Build history of the part. All positions in model axes, mm. Face numbers are marked on the shaded views. A direction names the side the tool comes from. Round coordinates to 2 decimals unless told otherwise and drop trailing zeros. Loops run counter-clockwise (first coordinate to the right, second up) from the corner with the lowest first, then second, coordinate; pieces in that order, holes last.
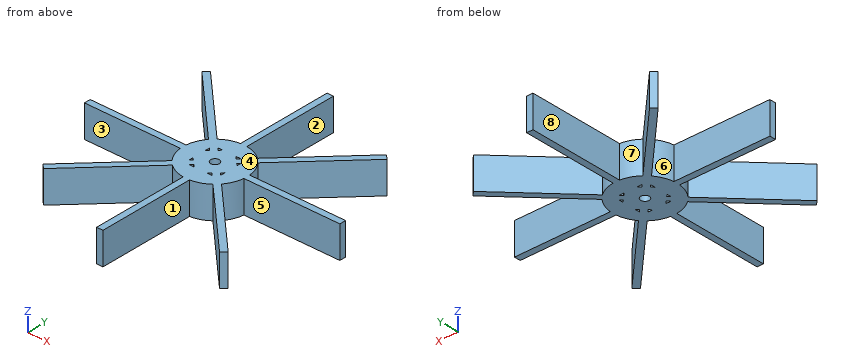
from build123d import *

# Parameters (mm, degrees)
F3_DEPTH = 10
F4_DEPTH = 10
F5_R     = 1.35
F6_DEPTH = 25


with BuildPart() as f3:
    # F2 (on Top) → F3 (new body)
    with BuildSketch(Plane.XY):
        Polygon((-2.9411380965, 1.5269245341), (-4.2426406871, 2.8284271247), (-7.0710678119, 0), (-5.7695652212, -1.3015025906), align=None)
        Polygon((-28.9913780286, 27.5771644663), (-4.2426406871, 2.8284271247), (-3.5355339059, 3.5355339059), (-2.8284271247, 4.2426406871), (-27.5771644663, 28.9913780286), align=None)
        Polygon((-3.5355339059, 3.5355339059), (-4.2426406871, 2.8284271247), (-2.9411380965, 1.5269245341), (-5.7695652212, -1.3015025906), (-4.2426406871, -2.8284271247), (-3.5355339059, -3.5355339059), (0, 0), align=None)
        Polygon((-2.8284271247, 4.2426406871), (-3.5355339059, 3.5355339059), (0, 0), (3.5355339059, 3.5355339059), (2.8284271247, 4.2426406871), (2.4045457253, 4.6665220865), (-0.4238813994, 1.8380949618), align=None)
        Polygon((0, 7.0710678119), (-2.8284271247, 4.2426406871), (-0.4238813994, 1.8380949618), (2.4045457253, 4.6665220865), align=None)
        Polygon((3.5355339059, 3.5355339059), (0, 0), (3.5355339059, -3.5355339059), (4.2426406871, -2.8284271247), (7.0710678119, 0), (4.2426406871, 2.8284271247), align=None)
        Polygon((3.5355339059, -3.5355339059), (0, 0), (-3.5355339059, -3.5355339059), (-2.8284271247, -4.2426406871), (0, -7.0710678119), (2.8284271247, -4.2426406871), align=None)
        Polygon((-3.5355339059, -3.5355339059), (-4.2426406871, -2.8284271247), (-28.9913780286, -27.5771644663), (-27.5771644663, -28.9913780286), (-2.8284271247, -4.2426406871), align=None)
        Polygon((4.2426406871, -2.8284271247), (3.5355339059, -3.5355339059), (2.8284271247, -4.2426406871), (27.5771644663, -28.9913780286), (28.9913780286, -27.5771644663), align=None)
        Polygon((2.8284271247, 4.2426406871), (3.5355339059, 3.5355339059), (4.2426406871, 2.8284271247), (28.9913780286, 27.5771644663), (27.5771644663, 28.9913780286), align=None)
    extrude(amount=F3_DEPTH)

    # F1 (on Top) → F4 (join)
    with BuildSketch(Plane.XY):
        with BuildLine():
            ThreePointArc((9.9498743711, -1), (9.9874607311, -0.5006277506), (10, 0))
            ThreePointArc((10, 0), (9.9874607311, 0.5006277506), (9.9498743711, 1))
            Line((9.9498743711, 1), (5, 1))
            Line((5, 1), (5, 0))
            Line((5, 0), (5, -1))
            Line((5, -1), (9.9498743711, -1))
        make_face()
        with BuildLine():
            ThreePointArc((9.9498743711, 1), (9.9874607311, 0.5006277506), (10, 0))
            ThreePointArc((10, 0), (9.9874607311, -0.5006277506), (9.9498743711, -1))
            Line((9.9498743711, -1), (40, -1))
            Line((40, -1), (40, 1))
            Line((40, 1), (9.9498743711, 1))
        make_face()
        with BuildLine():
            Line((5, 1), (9.9498743711, 1))
            ThreePointArc((9.9498743711, 1), (7.0710678119, 7.0710678119), (1, 9.9498743711))
            Line((1, 9.9498743711), (1, 5))
            Line((1, 5), (5, 5))
            Line((5, 5), (5, 1))
        make_face()
        with BuildLine():
            ThreePointArc((1, -9.9498743711), (7.0710678119, -7.0710678119), (9.9498743711, -1))
            Line((9.9498743711, -1), (5, -1))
            Line((5, -1), (5, -5))
            Line((5, -5), (1, -5))
            Line((1, -5), (1, -9.9498743711))
        make_face()
        with BuildLine():
            Line((1, 5), (1, 9.9498743711))
            ThreePointArc((1, 9.9498743711), (0, 10), (-1, 9.9498743711))
            Line((-1, 9.9498743711), (-1, 5))
            Line((-1, 5), (0, 5))
            Line((0, 5), (1, 5))
        make_face()
        with BuildLine():
            ThreePointArc((-1, 9.9498743711), (0, 10), (1, 9.9498743711))
            Line((1, 9.9498743711), (1, 40))
            Line((1, 40), (-1, 40))
            Line((-1, 40), (-1, 9.9498743711))
        make_face()
        with BuildLine():
            Line((1, -40), (1, -9.9498743711))
            ThreePointArc((1, -9.9498743711), (0, -10), (-1, -9.9498743711))
            Line((-1, -9.9498743711), (-1, -40))
            Line((-1, -40), (1, -40))
        make_face()
        with BuildLine():
            ThreePointArc((-1, -9.9498743711), (0, -10), (1, -9.9498743711))
            Line((1, -9.9498743711), (1, -5))
            Line((1, -5), (-1, -5))
            Line((-1, -5), (-1, -9.9498743711))
        make_face()
        with BuildLine():
            Line((-1, 5), (-1, 9.9498743711))
            ThreePointArc((-1, 9.9498743711), (-7.0710678119, 7.0710678119), (-9.9498743711, 1))
            Line((-9.9498743711, 1), (-5, 1))
            Line((-5, 1), (-5, 5))
            Line((-5, 5), (-1, 5))
        make_face()
        with BuildLine():
            ThreePointArc((-9.9498743711, -1), (-7.0710678119, -7.0710678119), (-1, -9.9498743711))
            Line((-1, -9.9498743711), (-1, -5))
            Line((-1, -5), (-5, -5))
            Line((-5, -5), (-5, -1))
            Line((-5, -1), (-9.9498743711, -1))
        make_face()
        with BuildLine():
            Line((-5, 1), (-9.9498743711, 1))
            ThreePointArc((-9.9498743711, 1), (-10, 0), (-9.9498743711, -1))
            Line((-9.9498743711, -1), (-5, -1))
            Line((-5, -1), (-5, 0))
            Line((-5, 0), (-5, 1))
        make_face()
        with BuildLine():
            ThreePointArc((-9.9498743711, -1), (-10, 0), (-9.9498743711, 1))
            Line((-9.9498743711, 1), (-40, 1))
            Line((-40, 1), (-40, -1))
            Line((-40, -1), (-9.9498743711, -1))
        make_face()
    extrude(amount=F4_DEPTH)

    # F5 (on face) → F6 (cut)
    with BuildSketch(Plane.XY.offset(10)):
        Circle(F5_R)
    extrude(amount=-F6_DEPTH, mode=Mode.SUBTRACT)


solid = f3.part
(1) Slice it at A-A on y = 0. List the corners of the cut face in (x, z), plus the area to 3 significant figures.
Responses:
outline: (-40, 0) - (-1.35, 0) - (-1.35, 10) - (-40, 10) - close; (1.35, 0) - (40, 0) - (40, 10) - (1.35, 10) - close
area: 773 mm2
(2) Which spindle directions (+Z, -Z, +X, -X, +Y, -Y) get a long thin tool onto all of the face, cutting with end or side? Do the marked faces 1, 2, 3, 4 and 5. Say none if no direction does.
Responses:
face 1: +Z, -Z, -Y
face 2: +Z, -Z, +Y
face 3: +Z, -Z, -X
face 4: +Z, +X, -X, +Y, -Y
face 5: +Z, -Z, +X
(3) Pull direction Y, two halves, no side cores. Call the marked faces 6, 7 and 8: +Y half, -Y half, draft (parallel to the pull), parting line (faces both ways), or undercut.
Responses:
face 6: undercut
face 7: +Y half
face 8: draft
(4) Slice it at D-D on z = 7.75. Count the separate pieces of the cut face and the enclosed holes in it, plus the area to 3 significant figures.
Responses:
separate pieces: 1
enclosed holes: 9
area: 784 mm2
(5) Pin check, flat tips, straight feed: P1, Ø0.8, axis at y = 3, z = 5.5, coming from the +X side; P2, Ø0.5, axis at x = 2.5, z = 3.5, coming from the -Y side; P3, Ø2, axis at y = -11.5, z = 8.5, coming from the +X side. Stop position of each tip, or through.
Responses:
P1: stops at x = 9.66
P2: stops at y = -9.74
P3: stops at x = 13.91
(6) Probe line 1 (Y direction, x = 0, z = 7); line 2 (Y direction, x = 8.5, z = 2); line 3 (Y direction, x = -14, z = 1.75). List the from-to ranges inside material, lowest first.
Responses:
line 1: y = -40 to -1.35, 1.35 to 40
line 2: y = -9.91 to -7.09, -5.27 to 5.27, 7.09 to 9.91
line 3: y = -15.41 to -12.59, -1 to 1, 12.59 to 15.41
(7) Slice it at C-C on x = 14. List the corners of the cut face in (y, z), plus the area to 3 significant figures.
Responses:
outline: (-15.41, 0) - (-12.59, 0) - (-12.59, 10) - (-15.41, 10) - close; (-1, 0) - (1, 0) - (1, 10) - (-1, 10) - close; (12.59, 0) - (15.41, 0) - (15.41, 10) - (12.59, 10) - close
area: 76.6 mm2
